from build123d import *

# Parameters (mm, degrees)
SKETCH2_R               = 10
BOSS_EXTRUDE1_DEPTH     = 30
CUT_EXTRUDE1_START      = -10
SKETCH3_R               = 10
SKETCH3_R_2             = 7.5
CUT_EXTRUDE1_DEPTH      = 10
CUT_EXTRUDE3_DEPTH      = 10
CUT_EXTRUDE3_DEPTH_BACK = 10
SKETCH5_R               = 2
FILLET2_R               = 10
BOSS_EXTRUDE2_START     = -67.5
SKETCH7_R               = 10
BOSS_EXTRUDE2_DEPTH     = 67.5
SKETCH8_R               = 50
SKETCH8_R_2             = 10
CUT_EXTRUDE6_DEPTH      = 107.770782567
SKETCH9_R               = 7.5
CUT_EXTRUDE7_DEPTH      = 10
CUT_EXTRUDE8_DEPTH      = 10
CUT_EXTRUDE8_DEPTH_BACK = 10
SKETCH10_R              = 2


with BuildPart() as part:
    # Sketch1 → Revolve1 (revolve)
    with BuildSketch(Plane.XY):
        Polygon((50, 25), (0, 25), (0, 22.5), (45, 22.5), (45, -22.5), (0, -22.5), (0, -25), (50, -25), align=None)
    revolve(axis=Axis((0, -25, 0), (0, 1, 0)))

    # Sketch2 → Boss-Extrude1 (add)
    with BuildSketch(Plane(origin=(0, 25, 0), x_dir=(1, 0, 0), z_dir=(0, 1, 0))):
        with Locations(Location((0, 0, 0), (0, 0, 180))):
            Circle(SKETCH2_R)
    extrude(amount=BOSS_EXTRUDE1_DEPTH)

    # Sketch3 → Cut-Extrude1 (cut)
    with BuildSketch(Plane(origin=(0, 55, 0), x_dir=(1, 0, 0), z_dir=(0, 1, 0)).offset(CUT_EXTRUDE1_START)):
        with Locations(Location((0, 0, 0), (0, 0, 180))):
            Circle(SKETCH3_R)
        with Locations(Location((0, 0, 0), (0, 0, 180))):
            Circle(SKETCH3_R_2, mode=Mode.SUBTRACT)
    extrude(amount=CUT_EXTRUDE1_DEPTH, mode=Mode.SUBTRACT)

    # Sketch5 → Cut-Extrude3 (cut, two sides: drawn at the far end of the back side and taken through both)
    with BuildSketch(Plane(origin=(0, 0, 0), x_dir=(0, 0, -1), z_dir=(1, 0, 0)).offset(-CUT_EXTRUDE3_DEPTH_BACK)):
        with Locations(Location((0, 50, 0), (0, 0, 180))):
            Circle(SKETCH5_R)
    extrude(amount=CUT_EXTRUDE3_DEPTH + CUT_EXTRUDE3_DEPTH_BACK, mode=Mode.SUBTRACT)

    # Fillet2
    fillet2_edges = [part.edges().sort_by_distance(p)[0] for p in [
        (-50, 25, 0),
    ]]
    fillet(fillet2_edges, radius=FILLET2_R)

    # Sketch7 → Boss-Extrude2 (add)
    with BuildSketch(Plane(origin=(0, 45, 0), x_dir=(1, 0, 0), z_dir=(0, 1, 0)).offset(BOSS_EXTRUDE2_START)):
        with Locations(Location((0, 0, 0), (0, 0, 180))):
            Circle(SKETCH7_R)
    extrude(amount=BOSS_EXTRUDE2_DEPTH)

    # Sketch8 → Cut-Extrude6 (cut, through all)
    with BuildSketch(Plane(origin=(0, 55, 0), x_dir=(1, 0, 0), z_dir=(0, 1, 0))):
        Circle(SKETCH8_R)
        with Locations(Location((0, 0, 0), (0, 0, 180))):
            Circle(SKETCH8_R_2, mode=Mode.SUBTRACT)
    extrude(amount=-CUT_EXTRUDE6_DEPTH, mode=Mode.SUBTRACT)

    # Sketch9 → Cut-Extrude7 (cut)
    with BuildSketch(Plane.XZ.offset(25)):
        with Locations(Location((0, 0, 0), (0, 0, 180))):
            Circle(SKETCH9_R)
    extrude(amount=-CUT_EXTRUDE7_DEPTH, mode=Mode.SUBTRACT)

    # Sketch10 → Cut-Extrude8 (cut, two sides: drawn at the far end of the back side and taken through both)
    with BuildSketch(Plane(origin=(0, 0, 0), x_dir=(0, 0, -1), z_dir=(1, 0, 0)).offset(-CUT_EXTRUDE8_DEPTH_BACK)):
        with Locations(Location((0, -20, 0), (0, 0, 180))):
            Circle(SKETCH10_R)
    extrude(amount=CUT_EXTRUDE8_DEPTH + CUT_EXTRUDE8_DEPTH_BACK, mode=Mode.SUBTRACT)


solid = part.part
Build history of the part. All positions in model axes, mm. A direction names the side the tool comes from. Give positions to 0.01 mm unless a question says otherwise; leave off trailing zeros. Order: outer loops, then holes, each group sorted by start corner. A loop starts at its lowest first (then second) coordinate and runs counter-clockwise, first axis right, second up. Notation, with made-up numbers: M -36,77 L -2,77 A15 cw -2,102 Z; hole C 79.5,65.25 d2. An arc over 180 degrees is marked long. Put each result on its own line as item: value.
Item 1: Which spindle directions (+Z, -Z, +X, -X, +Y, -Y) get a long thin tool onto all of the face, cutting with end or side? Do faces 4 (the face through (-0.105, 51.774, 0.923)), 5 (the face through (-7.154, 49.93, 2.253)), 6 (the face through (-7.154, -20.07, -2.253)). Say none if no direction does.
Results are:
face 4: +X, -X
face 5: +Y
face 6: -Y
Item 2: Cut at A-A on z = 0. Write the cut outline in (x, y).
Results are:
outline: M -10,-25 L -7.5,-25 L -7.5,-22 L -10,-22 Z; M -10,-18 L -7.5,-18 L -7.5,-15 L 7.5,-15 L 7.5,-18 L 10,-18 L 10,45 L 7.5,45 L 7.5,48 L -7.5,48 L -7.5,45 L -10,45 Z; M -7.5,52 L 7.5,52 L 7.5,55 L -7.5,55 Z; M 7.5,-25 L 10,-25 L 10,-22 L 7.5,-22 Z
Item 3: Cut at D-D on y = 50. Write the cut outline in (x, z), then the cut area to 3 significant figures.
Results are:
outline: M -7.23,-2 A7.5 ccw 7.23,-2 Z; M -7.23,2 L 7.23,2 A7.5 ccw Z
area: 117 mm2
Item 4: Drop flat-ended pins along their axis: pin 1 Ø1.5 at (x, z) = (-0.5, 3.5) entering from -Y; pin 2 Ø1 at (y, z) = (18.5, -2) entering from +X; pin 3 Ø4 at (x, y) = (-3, 35.5) entering from -Z; pin 4 Ø3 at (y, z) = (-20, 0) entering from +X. Give the stop position or say it passes through.
Results are:
pin 1: y = -15
pin 2: x = 9.89
pin 3: z = -9.95
pin 4: through
Item 5: Wall check: probe 1 along Y at (x, z) = (-2, 0); probe 2 along Z at (x, y) = (0, -21); probe 3 along Y at (x, z) = (4.25, -5.25). Give the ranges that are in metal, low to high.
Results are:
probe 1: -15 to 48, 52 to 55
probe 2: -10 to -7.5, 7.5 to 10
probe 3: -15 to 55
Item 6: Pull direction Y, two halves, no side cores. Call faces 1 (the face through (-9, -20, -2)), 2 (the face through (-4, -25, -7)), 3 (the face through (0, 55, 0)): +Y half, -Y half, draft (parallel to the pull), parting line (faces both ways), or undercut.
Results are:
face 1: undercut
face 2: -Y half
face 3: +Y half
Item 7: Cut at C-C on y = -20. Write the cut outline in (x, z), then the cut area to 3 significant figures.
Results are:
outline: M -9.8,-2 A10 ccw 9.8,-2 L 7.23,-2 A7.5 cw -7.23,-2 Z; M -9.8,2 L -7.23,2 A7.5 cw 7.23,2 L 9.8,2 A10 ccw Z
area: 117 mm2
Item 8: Cut at B-B on x = 0. Write the cut outline in (y, z).
Results are:
outline: M -25,-10 L 45,-10 L 45,-7.5 L 55,-7.5 L 55,7.5 L 45,7.5 L 45,10 L -25,10 L -25,7.5 L -15,7.5 L -15,-7.5 L -25,-7.5 Z; hole C 50,0 d4
